Read the model definition and answer for the solid it produces. Units are mm, in the model's axes. A direction names the side the tool comes from. Round coordinates to 2 decimals unless told otherwise and drop trailing zeros. Write each loop counter-clockwise with the first axis right and the second up, starting at its lowest first coordinate (ties: lowest second). Pieces come first, ordered by that corner, then holes. Notation, with made-up numbers: M 24,-4.75 L 52,-4.75 A25 ccw 52,23.25 Z; hole C -36,1 d9. An arc over 180 degrees is marked long. Use one line per item in the form item = value. Start each with the question number.
```python
from build123d import *

# Parameters (mm, degrees)
SKETCH1_W           = 9.525
SKETCH1_H           = 44.45
BOSS_EXTRUDE1_DEPTH = 12.7
SKETCH2_R           = 3.429
CUT_EXTRUDE1_DEPTH  = 6.35
SKETCH3_R           = 1.397
CUT_EXTRUDE2_DEPTH  = 33.348528515
SKETCH4_R           = 4.826
SKETCH4_R_2         = 4.7625
CUT_EXTRUDE3_DEPTH  = 35.841784793


with BuildPart() as part:
    # Sketch1 → Boss-Extrude1 (new body)
    with BuildSketch(Plane.XY):
        with Locations((-1.883585653, 8.79006638)):
            Rectangle(SKETCH1_W, SKETCH1_H)
    extrude(amount=BOSS_EXTRUDE1_DEPTH)

    # Sketch2 → Cut-Extrude1 (cut)
    with BuildSketch(Plane.XY.offset(12.7)):
        with Locations((-1.883585653, 27.11616638)):
            Circle(SKETCH2_R)
        with Locations((-1.883585653, -9.53603362)):
            Circle(SKETCH2_R)
    extrude(amount=-CUT_EXTRUDE1_DEPTH, mode=Mode.SUBTRACT)

    # Sketch3 → Cut-Extrude2 (cut, through all)
    with BuildSketch(Plane.XY.offset(6.35)):
        with Locations((-1.883585653, 27.11616638)):
            Circle(SKETCH3_R)
        with Locations((-1.883585653, -9.53603362)):
            Circle(SKETCH3_R)
    extrude(amount=-CUT_EXTRUDE2_DEPTH, mode=Mode.SUBTRACT)

    # Sketch4 → Cut-Extrude3 (cut, through all)
    with BuildSketch(Plane.ZY.offset(6.646085653)):
        with Locations((1.312301335, -0.841200319)):
            Circle(SKETCH4_R)
        with Locations((1.312301335, -0.841200319)):
            Circle(SKETCH4_R_2, mode=Mode.SUBTRACT)
    extrude(amount=-CUT_EXTRUDE3_DEPTH, mode=Mode.SUBTRACT)


with BuildPart() as cut_extrude3_kept_piece:
    # of the separate pieces the step leaves, the one the design keeps (cut_extrude3_pieces_kept)
    add(part.part.solids().sort_by_distance((-6.646085653, 31.01506638, 0))[0])


solid = cut_extrude3_kept_piece.part
```
Q1. A tool of negligible diameter and unlimited length cuts with its end or side. For faces 1 (the face through (-2.33, -6.136, 9.569)), 2 (the face through (-2, -13.435, 6)), from which of +Z, -Z, +X, -X, +Y, -Y can it reach the whole face along a straight path? Write none if from no direction.
Q2. For a pull along Z with two mould halves and no side action, classify faces 3 (the face through (-2, 18, 0)), 4 (the face through (-1.95, -0.966, 6.137)), 5 (the face through (0, 27, 6.35)), 6 (the face through (-2.63, 23.77, 9.57)) as +Z half, -Z half, draft (parallel to the pull), parting line (faces both ways), or undercut.
Q3. Straight lines are drawn through the part: line 1 (Y direction, x = -3, z = 1.25); line 2 (Y direction, x = -3.5, z = 12.25); line 3 (X direction, y = 27, z = 11.75). For each, find the intervals that lie inside material, in ascending order. Write a range as [from, to].
Q4. Find section C-C on y = -10. Write down the section's boundary in (x, z), and give its area (3 significant figures).
Q5. Find section D-D on z = 5.75. Write down the section's boundary in (x, y).
Q6. Find section B-B on x = -1. Write down the section's boundary in (y, z).
Q7. Each of these flat-tipped pins is pushed along its axis until it touches: pin 1 Ø2 at (x, y) = (-0.5, 26) entering from +Z; pin 2 Ø1.7 at (x, y) = (-1.88, 27.12) entering from +Z. Where does it stop, or does it pass through?
Q8. Find section A-A on z = 3.25. Write down the section's boundary in (x, y), and give its area (3 significant figures).
Response:
q1.face_1 = +Z
q1.face_2 = +Z, -Z, +X, -X, -Y
q2.face_3 = -Z half
q2.face_4 = undercut
q2.face_5 = +Z half
q2.face_6 = draft
q3.line_1 = [-13.43, -10.38], [-8.7, -5.67], [3.98, 26.28], [27.96, 31.02]
q3.line_2 = [-13.43, -12.56], [-6.51, 24.09], [30.14, 31.02]
q3.line_3 = [-6.65, -5.31], [1.54, 2.88]
q4.outline = M -6.65,0 L -3.2,0 L -3.2,6.35 L -5.28,6.35 L -5.28,12.7 L -6.65,12.7 Z; M -0.57,0 L 2.88,0 L 2.88,12.7 L 1.51,12.7 L 1.51,6.35 L -0.57,6.35 Z
q4.area = 61.1 mm²
q5.outline = M -6.65,-13.43 L 2.88,-13.43 L 2.88,-2.74 L -6.65,-2.74 Z; M -6.65,1.06 L 2.88,1.06 L 2.88,31.02 L -6.65,31.02 Z; hole C -1.88,-9.54 d2.79; hole C -1.88,27.12 d2.79
q6.outline = M -13.43,0 L -10.62,0 L -10.62,6.35 L -12.85,6.35 L -12.85,12.7 L -13.43,12.7 Z; M -8.45,0 L -5.49,0 A4.83 cw long 3.8,0 L 26.03,0 L 26.03,6.35 L 23.8,6.35 L 23.8,12.7 L -6.22,12.7 L -6.22,6.35 L -8.45,6.35 Z; M 28.2,0 L 31.02,0 L 31.02,12.7 L 30.43,12.7 L 30.43,6.35 L 28.2,6.35 Z
q7.pin_1 = 6.35
q7.pin_2 = through
q8.outline = M -6.65,-13.43 L 2.88,-13.43 L 2.88,-5.26 L -6.65,-5.26 Z; M -6.65,3.58 L 2.88,3.58 L 2.88,31.02 L -6.65,31.02 Z; hole C -1.88,-9.54 d2.79; hole C -1.88,27.12 d2.79
q8.area = 327 mm²
